from build123d import *

# Parameters (mm, degrees)
BOSS_EXTRUDE1_DEPTH      = 12.5
BOSS_EXTRUDE1_DEPTH_BACK = 12.5
SKETCH1_W                = 25
SKETCH1_H                = 25
SKETCH1_W_2              = 23
SKETCH1_H_2              = 23
SKETCH2_R                = 2
CUT_EXTRUDE1_DEPTH       = 25
SKETCH3_R                = 1.5
CUT_EXTRUDE2_DEPTH       = 25


with BuildPart() as part:
    # Sketch1 → Boss-Extrude1 (new, two sides: drawn at the far end of the back side and taken through both)
    with BuildSketch(Plane(origin=(0, 0, 0), x_dir=(1, 0, 0), z_dir=(0, 1, 0)).offset(-BOSS_EXTRUDE1_DEPTH_BACK)):
        Rectangle(SKETCH1_W, SKETCH1_H)
        Rectangle(SKETCH1_W_2, SKETCH1_H_2, mode=Mode.SUBTRACT)
    extrude(amount=BOSS_EXTRUDE1_DEPTH + BOSS_EXTRUDE1_DEPTH_BACK)

    # Sketch2 → Cut-Extrude1 (cut)
    with BuildSketch(Plane(origin=(0, 0, -12.5), x_dir=(-1, 0, 0), z_dir=(0, 0, -1))):
        with Locations((5.5, 5.5)):
            Circle(SKETCH2_R)
        with Locations((5.5, -5.5)):
            Circle(SKETCH2_R)
        with Locations((-5.5, -5.5)):
            Circle(SKETCH2_R)
        with Locations((-5.5, 5.5)):
            Circle(SKETCH2_R)
    extrude(amount=-CUT_EXTRUDE1_DEPTH, mode=Mode.SUBTRACT)

    # Sketch3 → Cut-Extrude2 (cut)
    with BuildSketch(Plane(origin=(12.5, 0, 0), x_dir=(0, 0, -1), z_dir=(1, 0, 0))):
        Circle(SKETCH3_R)
    extrude(amount=-CUT_EXTRUDE2_DEPTH, mode=Mode.SUBTRACT)


solid = part.part
CAD build for the part. Positions are in the model's coordinates, mm. A direction names the side the tool comes from. Give positions to 0.01 mm unless a question says otherwise; leave off trailing zeros. Loops run counter-clockwise (first coordinate to the right, second up) from the corner with the lowest first, then second, coordinate; pieces in that order, holes last. Notation, with made-up numbers: M 18.5,-6.75 L 30.5,-6.75 A26 ccw 30.5,20.25 Z; hole C -13.5,81 d9. An arc over 180 degrees is marked long. Answer in a Markdown table with one row per item. Add a question column.
Item 1: Probe probe 1 along Y at (x, z) = (5.5, -12.15); probe 2 along Z at (x, y) = (7.5, 11.25). List the from-to ranges inside material, lowest first.
Item 2: Band-saw the part on A-A on z = 0. Give the cut face in (x, y).
Item 3: Band-saw the part on B-B on y = 5.5. Give the cut face in (x, z), then the cut area to 3 significant figures.
Item 4: Mould opens along Z. For faces 1 (the face through (-12.5, -3, 0)), 2 (the face through (0, 0, 11.5)), 3 (the face through (0, 0, -11.5)), 4 (the face through (0, 0, 12.5)) say: +Z half, -Z half, draft (parallel to the pull), parting line (faces both ways), or undercut.
Item 5: Tool access for faces 5 (the face through (11.5, 0, 3)), 6 (the face through (7.1, -6.7, 12)): list every direction of +Z, -Z, +X, -X, +Y, -Y with a clear straight run to the whole face (end or side of a thin tool).
Item 6: Band-saw the part on D-D on y = -2.5. Give the cut face in (x, z), then the cut area to 3 significant figures.
Item 7: Band-saw the part on C-C on x = -5.5. Give the cut face in (y, z).
Item 8: Drop a flat-ended pin along its axis: P1, Ø5, axis at x = 5.5, y = 5.5, coming from the -Z side. Give the stop position or say it passes through.
Reply:
| question | item | result |
|---|---|---|
| 1 | probe 1 | y = -12.5 to -7.5, -3.5 to 3.5, 7.5 to 12.5 |
| 1 | probe 2 | z = -12.5 to -11.5, 11.5 to 12.5 |
| 2 | outline | M -12.5,-12.5 L -11.5,-12.5 L -11.5,-1.5 L -12.5,-1.5 Z; M -12.5,1.5 L -11.5,1.5 L -11.5,12.5 L -12.5,12.5 Z; M 11.5,-12.5 L 12.5,-12.5 L 12.5,-1.5 L 11.5,-1.5 Z; M 11.5,1.5 L 12.5,1.5 L 12.5,12.5 L 11.5,12.5 Z |
| 3 | outline | M -12.5,-12.5 L -7.5,-12.5 L -7.5,-11.5 L -11.5,-11.5 L -11.5,11.5 L -7.5,11.5 L -7.5,12.5 L -12.5,12.5 Z; M -3.5,-12.5 L 3.5,-12.5 L 3.5,-11.5 L -3.5,-11.5 Z; M -3.5,11.5 L 3.5,11.5 L 3.5,12.5 L -3.5,12.5 Z; M 7.5,-12.5 L 12.5,-12.5 L 12.5,12.5 L 7.5,12.5 L 7.5,11.5 L 11.5,11.5 L 11.5,-11.5 L 7.5,-11.5 Z |
| 3 | area | 80.0 mm^2 |
| 4 | face 1 | draft |
| 4 | face 2 | undercut |
| 4 | face 3 | undercut |
| 4 | face 4 | +Z half |
| 5 | face 5 | +Y, -Y |
| 5 | face 6 | +Z, -Z |
| 6 | outline | M -12.5,-12.5 L 12.5,-12.5 L 12.5,12.5 L -12.5,12.5 Z; hole M -11.5,-11.5 L 11.5,-11.5 L 11.5,11.5 L -11.5,11.5 Z |
| 6 | area | 96.0 mm^2 |
| 7 | outline | M -12.5,-12.5 L -7.5,-12.5 L -7.5,-11.5 L -12.5,-11.5 Z; M -12.5,11.5 L -7.5,11.5 L -7.5,12.5 L -12.5,12.5 Z; M -3.5,-12.5 L 3.5,-12.5 L 3.5,-11.5 L -3.5,-11.5 Z; M -3.5,11.5 L 3.5,11.5 L 3.5,12.5 L -3.5,12.5 Z; M 7.5,-12.5 L 12.5,-12.5 L 12.5,-11.5 L 7.5,-11.5 Z; M 7.5,11.5 L 12.5,11.5 L 12.5,12.5 L 7.5,12.5 Z |
| 8 | P1 | stops at z = -12.5 |
